from build123d import *

# Parameters (mm, degrees)
SKETCH2_W           = 100
SKETCH2_H           = 100
BOSS_EXTRUDE1_DEPTH = 30
BOSS_EXTRUDE2_DEPTH = 10
SKETCH5_R           = 4.25
CUT_EXTRUDE1_DEPTH  = 15
CHAMFER1_SIZE       = 0.85
SKETCH7_R           = 4
CUT_EXTRUDE2_DEPTH  = 15
CHAMFER2_SIZE       = 0.1


with BuildPart() as part:
    # Sketch2 → Boss-Extrude1 (new body)
    with BuildSketch(Plane(origin=(0, 0, 0), x_dir=(1, 0, 0), z_dir=(0, 1, 0))):
        Rectangle(SKETCH2_W, SKETCH2_H)
    extrude(amount=BOSS_EXTRUDE1_DEPTH)

    # Sketch4 → Boss-Extrude2 (add)
    with BuildSketch(Plane(origin=(0, 30, 0), x_dir=(1, 0, 0), z_dir=(0, 1, 0))):
        with BuildLine():
            Line((-50, -50), (-50, 0))
            Line((-50, 0), (0, 0))
            ThreePointArc((0, 0), (4.330127019, -7.5), (-4.330127019, -7.5))
            ThreePointArc((-4.330127019, -7.5), (-6.160254038, -5.669872981), (-8.660254038, -5))
            Line((-8.660254038, -5), (-15, -5))
            ThreePointArc((-15, -5), (-18.535533906, -6.464466094), (-20, -10))
            Line((-20, -10), (-20, -50))
            Line((-20, -50), (-50, -50))
        make_face()
    extrude(amount=BOSS_EXTRUDE2_DEPTH)

    # Sketch5 → Cut-Extrude1 (cut)
    with BuildSketch(Plane(origin=(0, 30, 0), x_dir=(1, 0, 0), z_dir=(0, 1, 0))):
        with Locations(Location((35, 35, 0), (0, 0, 270))):
            Circle(SKETCH5_R)
        with Locations(Location((-35, 35, 0), (0, 0, 270))):
            Circle(SKETCH5_R)
        with Locations(Location((35, -35, 0), (0, 0, 270))):
            Circle(SKETCH5_R)
    extrude(amount=-CUT_EXTRUDE1_DEPTH, mode=Mode.SUBTRACT)

    # Chamfer1
    chamfer1_edges = [part.edges().sort_by_distance(p)[0] for p in [
        (35, 30, 30.75),
        (-35, 30, -39.25),
        (35, 30, -39.25),
    ]]
    chamfer(chamfer1_edges, length=CHAMFER1_SIZE)

    # Sketch7 → Cut-Extrude2 (cut)
    with BuildSketch(Plane(origin=(0, 40, 0), x_dir=(1, 0, 0), z_dir=(0, 1, 0))):
        with Locations(Location((-35, -35, 0), (0, 0, 270))):
            Circle(SKETCH7_R)
    extrude(amount=-CUT_EXTRUDE2_DEPTH, mode=Mode.SUBTRACT)

    # Chamfer2
    chamfer2_edges = [part.edges().sort_by_distance(p)[0] for p in [
        (-35, 40, 31),
    ]]
    chamfer(chamfer2_edges, length=CHAMFER2_SIZE)


solid = part.part
Input: part model. Units: mm. Frame: model coordinates. A direction names the side the tool comes from. Give positions to 0.01 mm unless a question says otherwise; leave off trailing zeros. Loops run counter-clockwise (first coordinate to the right, second up) from the corner with the lowest first, then second, coordinate; pieces in that order, holes last. Notation, with made-up numbers: (41, 87) - (70, 87) arc R24 cw to (70, 114) - close; hole circle Ø3 at (59, 46). An arc over 180 degrees is marked (long way). Use CSV: the item, a comma, the result in double quotes. Start each with the question number.
Item 1: Section C-C on z = 35. Return loops of the section in (x, y), then the cut area to 3 significant figures.
Item 2: Contact query for flat-ended pins moving along their axis: P1, Ø2.5, axis at x = -35, z = -33.5, coming from the +Y side; P2, Ø2.5, axis at x = -33.5, z = 33.5, coming from the +Y side; P3, Ø3, axis at x = -13, y = 36, coming from the +Z side. Output: stop coordinate, or through.
Item 3: Section A-A on y = 23.5. Return loops of the section in (x, z), then the cut area to 3 significant figures.
Item 4: Mould query, pull axis Z, two halves, no side actions, for faces 1 (the flat face through (35, 15, -35)), 2 (the flat face through (-25, 35, 0)), 3 (the flat face through (50, 15, 1)). Classes: pulls with the +Z half, pulls with the -Z half, needs draft (parallel to the pull), parting line crosses it, or undercut.
Item 5: Section D-D on y = 36. Return loops of the section in (x, z).
Item 6: Reachability of faces 4 (the flat face through (1, 15, 50)), 5 (the cylindrical face through (35.187, 22.174, -39.246)), 6 (the flat face through (-12, 35, 5)) from +Z, -Z, +X, -X, +Y, -Y: full face, straight path, thin tool, end or side. Return the list, or none.
Item 7: Section B-B on x = -35. Return loops of the section in (y, z).
Item 8: Line query: line 1 (X direction, y = 25, z = -35); line 2 (X direction, y = 20.75, z = 35); line 3 (Y direction, x = 14, z = -30.5). Output: solid intervals per line, ascending.
Ans:
1,outline,"(-50, 0) - (50, 0) - (50, 30) - (40.1, 30) - (39.25, 29.15) - (39.25, 15) - (30.75, 15) - (30.75, 29.15) - (29.9, 30) - (-20, 30) - (-20, 40) - (-30.9, 40) - (-31, 39.9) - (-31, 25) - (-39, 25) - (-39, 39.9) - (-39.1, 40) - (-50, 40) - close"
1,area,"3,050 mm2"
2,P1,"stops at y = 15"
2,P2,"stops at y = 25"
2,P3,"stops at z = 5"
3,outline,"(-50, -50) - (50, -50) - (50, 50) - (-50, 50) - close; hole circle Ø8.5 at (-35, -35); hole circle Ø8.5 at (35, -35); hole circle Ø8.5 at (35, 35)"
3,area,"9,830 mm2"
4,face 1,"undercut"
4,face 2,"pulls with the -Z half"
4,face 3,"needs draft"
5,outline,"(-50, 0) - (0, 0) arc R5 ccw (long way) to (-4.33, 7.5) arc R5 cw to (-8.66, 5) - (-15, 5) arc R5 cw to (-20, 10) - (-20, 50) - (-50, 50) - close; hole circle Ø8 at (-35, 35)"
6,face 4,"+Z, +X, -X, +Y, -Y"
6,face 5,"+Y"
6,face 6,"+Z, +Y"
7,outline,"(0, -50) - (30, -50) - (30, -40.1) - (29.15, -39.25) - (15, -39.25) - (15, -30.75) - (29.15, -30.75) - (30, -29.9) - (30, 0) - (40, 0) - (40, 30.9) - (39.9, 31) - (25, 31) - (25, 39) - (39.9, 39) - (40, 39.1) - (40, 50) - (0, 50) - close"
8,line 1,"x = -50 to -39.25, -30.75 to 30.75, 39.25 to 50"
8,line 2,"x = -50 to 30.75, 39.25 to 50"
8,line 3,"y = 0 to 30"
